Read the model definition and answer for the solid it produces. Units are mm, in the model's axes. Face numbers are marked on the shaded views. Give positions to 0.01 mm unless a question says otherwise; leave off trailing zeros. Write each loop counter-clockwise with the first axis right and the second up, starting at its lowest first coordinate (ties: lowest second). Pieces come first, ordered by that corner, then holes. Notation, with made-up numbers: M -8.75,82 L 0.25,82 A23 ccw 0.25,90 Z; hole C 35.5,70.5 d1. An arc over 180 degrees is marked long. Put each result on its own line as item: value.
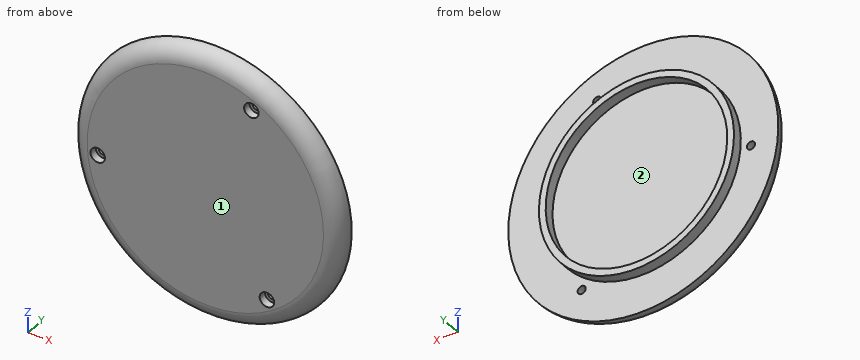
from build123d import *

# Parameters (mm, degrees)
SKETCH_1_R                = 40
EXTRUDE_1_DEPTH           = 5
SKETCH_2_R                = 28.9
EXTRUDE_2_DEPTH           = 3
HOLE_WIZARD_1_D           = 2.4
HOLE_WIZARD_1_CBORE_D     = 4.3
HOLE_WIZARD_1_CBORE_DEPTH = 2.3
PATTERN_CIRCULAR_1_COUNT  = 3
SKETCH_7_R                = 26.9
CUT_EXTRUDE_1_DEPTH       = 3
FILLET_1_R                = 5


with BuildPart() as part:
    # 草图1 → 凸台-拉伸1 (new body)
    with BuildSketch(Plane(origin=(0, 0, 0), x_dir=(1, 0, 0), z_dir=(0, 1, 0))):
        with Locations(Location((0, 0, 0), (0, 0, 270))):
            Circle(SKETCH_1_R)
    extrude(amount=EXTRUDE_1_DEPTH)

    # 草图2 → 凸台-拉伸2 (add)
    with BuildSketch(Plane(origin=(0, 5, 0), x_dir=(1, 0, 0), z_dir=(0, 1, 0))):
        with Locations(Location((0, 0, 0), (0, 0, 270))):
            Circle(SKETCH_2_R)
    extrude(amount=EXTRUDE_2_DEPTH)

    # 打孔尺寸(%根据)内六角圆柱头螺钉的类型1 (through all)
    with Locations(Plane(origin=(0, 0, 0), x_dir=(-1, 0, 0), z_dir=(0, -1, 0))):
        with Locations((-13.645026716, -28.945003816)):
            hole_wizard_1 = CounterBoreHole(HOLE_WIZARD_1_D / 2, HOLE_WIZARD_1_CBORE_D / 2, HOLE_WIZARD_1_CBORE_DEPTH)

    # 阵列(圆周)1: 打孔尺寸(%根据)内六角圆柱头螺钉的类型1 ×3 about axis
    pattern_circular_1_axis = Axis((0, 0, 0), (0, 1, 0))
    for i in range(1, PATTERN_CIRCULAR_1_COUNT):
        add(hole_wizard_1.rotate(pattern_circular_1_axis, i * 360 / PATTERN_CIRCULAR_1_COUNT), mode=Mode.SUBTRACT)

    # 草图7 → 切除-拉伸1 (cut)
    with BuildSketch(Plane(origin=(0, 8, 0), x_dir=(1, 0, 0), z_dir=(0, 1, 0))):
        with Locations(Location((0, 0, 0), (0, 0, 270))):
            Circle(SKETCH_7_R)
    extrude(amount=-CUT_EXTRUDE_1_DEPTH, mode=Mode.SUBTRACT)

    # 圆角1
    fillet_1_edges = [part.edges().sort_by_distance(p)[0] for p in [
        (0, 0, -40),
    ]]
    fillet(fillet_1_edges, radius=FILLET_1_R - 0.0001)  # a hair under: the kernel refuses the full size


solid = part.part
(1) Straight lines are drawn through the part: line 1 along X through (y, z) = (6, 0); line 2 along Y through (x, z) = (6.5, -17); line 3 along X through (y, z) = (5.25, 9). For each, find the intervals that lie inside material, in ascending order. Write a range as from..to.
Result:
line 1: x = -28.9..-26.9, 26.9..28.9
line 2: y = 0..5
line 3: x = -27.46..-25.35, 25.35..27.46
(2) For a pull along Z with two mould halves and no side action, classify the marked faces 1 and 2 as +Z half, -Z half, draft (parallel to the pull), parting line (faces both ways), or undercut.
Result:
face 1: draft
face 2: undercut
(3) Given pin 1 Ø1.3 at (x, z) = (18, -27) entering from -Y; pin 2 Ø4 at (x, z) = (6.5, 17.5) entering from +Y; pin 3 Ø12 at (x, z) = (30.5, -29) entering from -Y, each flat-ended and moving along its own axis, determine where each tip first touches the part or whether it passes through.
Result:
pin 1: stops at y = 2.3
pin 2: stops at y = 5
pin 3: stops at y = 0.12
(4) Section C-C on y = 1.25 is taken. Give the number of separate pieces and of enclosed holes in the cut face, and give its area (3 significant figures).
Result:
separate pieces: 1
enclosed holes: 3
area: 4,570 mm²
(5) Section B-B on y = 7 is taken. Determine the outline of the cut face in (x, z), and give its area (3 significant figures).
Result:
outline: C 0,0 d57.8; hole C 0,0 d53.8
area: 351 mm²
